from build123d import *

# Parameters (mm, degrees)
F2_W     = 603
F2_H     = 535
F2_R     = 10
F2_R_2   = 201
F3_DEPTH = 10
F4_W     = 493
F4_H     = 10
F4_W_2   = 10
F4_H_2   = 535
F5_DEPTH = 50


with BuildPart() as f1:
    # F0 (on Front) → F1 (revolve)
    with BuildSketch(Plane.XZ):
        Polygon((-201, -100), (-200, -100), (-200, 55), (-201, 55), (-201, 95), (-249, 95), (-249, 55), (-250, 55), (-250, -100), (-249, -100), (-249, -60), (-201, -60), align=None)
    revolve(axis=Axis((0, 0, -77.049306), (0, 0, -1)))

    # F2 (on Top) → F3 (join)
    with BuildSketch(Plane.XY):
        Rectangle(F2_W, F2_H)
        with Locations((-271.5, -237.5)):
            Circle(F2_R, mode=Mode.SUBTRACT)
        with Locations((271.5, -237.5)):
            Circle(F2_R, mode=Mode.SUBTRACT)
        with Locations((-271.5, 237.5)):
            Circle(F2_R, mode=Mode.SUBTRACT)
        Circle(F2_R_2, mode=Mode.SUBTRACT)
        with Locations((271.5, 237.5)):
            Circle(F2_R, mode=Mode.SUBTRACT)
    extrude(amount=-F3_DEPTH)

    # F4 (on face) → F5 (join)
    with BuildSketch(Plane(origin=(0, 0, -10), x_dir=(1, 0, 0), z_dir=(0, 0, -1))):
        with Locations((0, 262.5)):
            Rectangle(F4_W, F4_H)
        with Locations((-296.5, 0)):
            Rectangle(F4_W_2, F4_H_2)
        with Locations((0, -262.5)):
            Rectangle(F4_W, F4_H)
        with Locations((296.5, 0)):
            Rectangle(F4_W_2, F4_H_2)
    extrude(amount=-F5_DEPTH)


solid = f1.part
Input: part model. Units: mm. Frame: model coordinates. A direction names the side the tool comes from. Give positions to 0.01 mm unless a question says otherwise; leave off trailing zeros. Write each loop counter-clockwise with the first axis right and the second up, starting at its lowest first coordinate (ties: lowest second). Pieces come first, ordered by that corner, then holes. Notation, with made-up numbers: (43, 4.5) -> (98, 4.5) arc R18 cw to (98, 35.5) -> close; hole circle Ø9 at (62.25, 31.5). An arc over 180 degrees is marked (long way). Use one line per item in the form item = value. Start each with the question number.
1) Set-up query: faces 4 (the cylindrical face through (-108.06, 169.48, 75.28)), 5 (the flat face through (291.5, 4, 20)), 6 (the flat face through (-17, 204, -60)), 7 (the flat face through (17, 204, 95)), 8 (the cylindrical face through (-278.87, -230.74, -4.93)). Return all of +Z, -Z, +X, -X, +Y, -Y with unobstructed straight access to the full face (end or side cutting, diameter ignored); none if empty.
2) Section query C-C on z = -86. Return the cut outline in (x, y), then the cut area to 3 significant figures.
3) Section query D-D on y = -237.5. Count the separate pieces of the cut face and the enclosed holes in it, then the cut area to 3 significant figures.
4) Pin query (flat end, axial travel): pin 1 (6 mm diameter, centred on x = 211, z = -14, fed in from -Y); pin 2 (5 mm diameter, centred on x = -296, y = -74.5, fed in from +Z); pin 3 (4 mm diameter, centred on y = -40, z = -72.5, fed in from +X). Return the tip coordinate at first contact, or that it passes through.
5) Draft query along Y for faces 1 (the cylindrical face through (-114.898, -220.906, 74.72)), 2 (the flat face through (-301.5, -4, 15)), 3 (the flat face through (-88, -237, 0)). Return one class per face: pulls with the +Y half, pulls with the -Y half, needs draft (parallel to the pull), parting line crosses it, or undercut.
6) Section query A-A on x = 271.5. Return the cut outline in (y, z), then the cut area to 3 significant figures.
7) Section query B-B on z = 15. Return the cut outline in (x, y), then the cut area to 3 significant figures.
8) Ray query, probe 1 along X at (y, z) = (237, -7); probe 2 along Y at (x, z) = (271, -3); probe 3 along X at (y, z) = (4.5, -72.5). Return the intervals inside material, ascending. Write a range as from..to.
Outcome:
q1.face_4 = +Z
q1.face_5 = +Z, +Y, -Y
q1.face_6 = -Z
q1.face_7 = +Z, +X, -X, +Y, -Y
q1.face_8 = +Z, -Z
q2.outline = circle Ø500 at (0, 0); circle Ø402 at (0, 0); hole circle Ø498 at (0, 0); hole circle Ø400 at (0, 0)
q2.area = 2,830 mm^2
q3.separate_pieces = 3
q3.enclosed_holes = 0
q3.area = 29,100 mm^2
q4.pin_1 = -138.69
q4.pin_2 = 40
q4.pin_3 = 247.1
q5.face_1 = parting line crosses it
q5.face_2 = needs draft
q5.face_3 = undercut
q6.outline = (-267.5, -10) -> (-247.5, -10) -> (-247.5, 0) -> (-267.5, 0) -> close; (-227.5, -10) -> (227.5, -10) -> (227.5, 0) -> (-227.5, 0) -> close; (247.5, -10) -> (267.5, -10) -> (267.5, 0) -> (247.5, 0) -> close
q6.area = 4,950 mm^2
q7.outline = (-301.5, -267.5) -> (-291.5, -267.5) -> (-291.5, 267.5) -> (-301.5, 267.5) -> close; circle Ø500 at (0, 0); (-246.5, -267.5) -> (246.5, -267.5) -> (246.5, -257.5) -> (-246.5, -257.5) -> close; (-246.5, 257.5) -> (246.5, 257.5) -> (246.5, 267.5) -> (-246.5, 267.5) -> close; (291.5, -267.5) -> (301.5, -267.5) -> (301.5, 267.5) -> (291.5, 267.5) -> close; hole circle Ø400 at (0, 0)
q7.area = 91,200 mm^2
q8.probe_1 = -301.5..-281.49, -261.51..261.51, 281.49..301.5
q8.probe_2 = -267.5..-247.49, -227.51..227.51, 247.49..267.5
q8.probe_3 = -249.96..-248.96, -200.95..-199.95, 199.95..200.95, 248.96..249.96
